Answer from the drawing. Dimensions are ordinates in mm from the lowest x, y and z of the part. A direction names the side the tool comes from. Coordinates: 2 decimals unless noted, no trailing zeros. Loops run counter-clockwise (first coordinate to the right, second up) from the corner with the lowest first, then second, coordinate; pieces in that order, holes last. Notation, with made-up numbers: M -0.5,4 L 9.5,4 A30 cw 9.5,34 Z; hole C -5,75.5 d8. An arc over 180 degrees is marked long. Put each result on its own line as item: value.
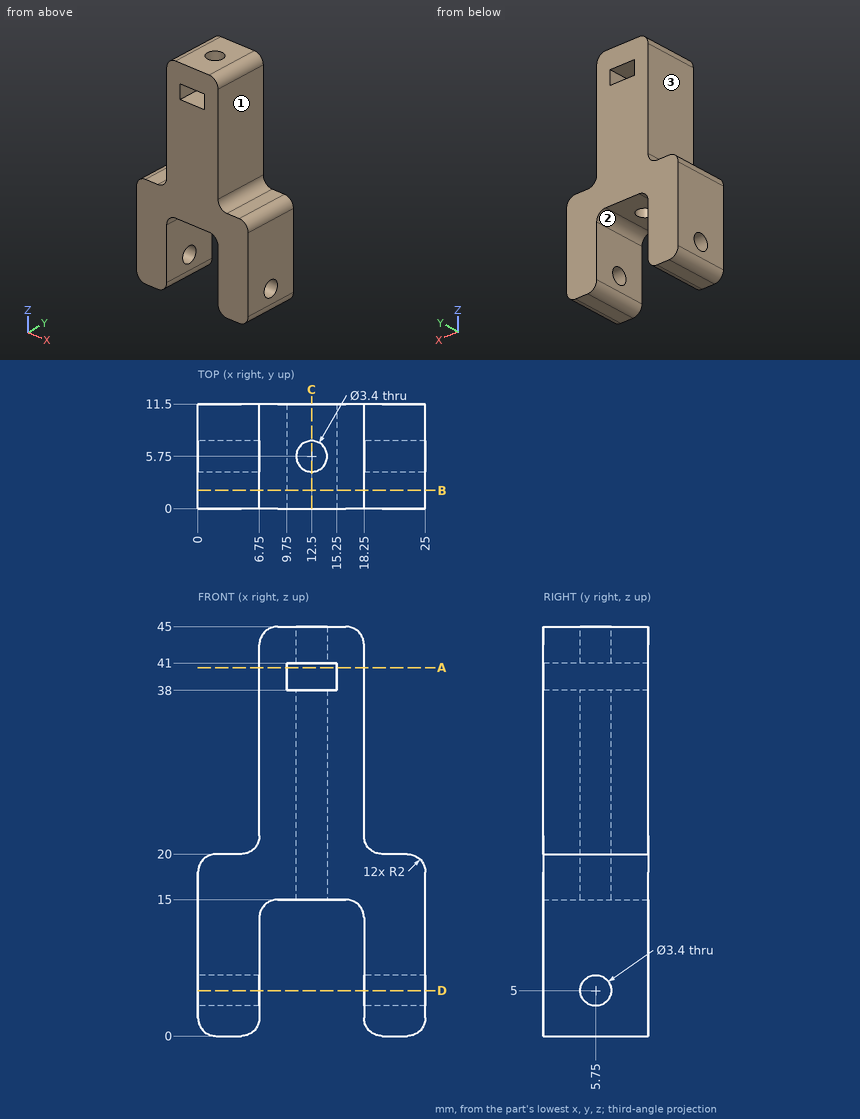
1) Find section B-B, the plane y = 2. Write down the section's boundary in (x, z).
Answer list:
outline: M 0,2 A2 ccw 2,0 L 4.75,0 A2 ccw 6.75,2 L 6.75,13 A2 cw 8.75,15 L 16.25,15 A2 cw 18.25,13 L 18.25,2 A2 ccw 20.25,0 L 23,0 A2 ccw 25,2 L 25,18 A2 ccw 23,20 L 20.25,20 A2 cw 18.25,22 L 18.25,43 A2 ccw 16.25,45 L 8.75,45 A2 ccw 6.75,43 L 6.75,22 A2 cw 4.75,20 L 2,20 A2 ccw 0,18 Z; hole M 9.75,38 L 15.25,38 L 15.25,41 L 9.75,41 Z
2) Given pin 1 Ø4.5 at (x, y) = (12.5, 5.75) entering from -Z; pin 2 Ø1.4 at (x, y) = (22, 3) entering from +Z; pin 3 Ø2.5 at (y, z) = (5, 40) entering from +X; pin 4 Ø3 at (y, z) = (5.75, 5) entering from -X, each flat-ended and moving along its own axis, determine where each tip first touches the part or whether it passes through.
Answer list:
pin 1: stops at z = 15
pin 2: stops at z = 20
pin 3: stops at x = 18.25
pin 4: passes through
3) Find section D-D, the plane z = 5. Write down the section's boundary in (x, y), plus the area to 3 significant figures.
Answer list:
outline: M 0,0 L 6.75,0 L 6.75,4.05 L 0,4.05 Z; M 0,7.45 L 6.75,7.45 L 6.75,11.5 L 0,11.5 Z; M 18.25,0 L 25,0 L 25,4.05 L 18.25,4.05 Z; M 18.25,7.45 L 25,7.45 L 25,11.5 L 18.25,11.5 Z
area: 109 mm^2
4) Find section C-C, the plane x = 12.5. Write down the section's boundary in (y, z), plus the area to 3 significant figures.
Answer list:
outline: M 0,15 L 4.05,15 L 4.05,38 L 0,38 Z; M 0,41 L 4.05,41 L 4.05,45 L 0,45 Z; M 7.45,15 L 11.5,15 L 11.5,38 L 7.45,38 Z; M 7.45,41 L 11.5,41 L 11.5,45 L 7.45,45 Z
area: 219 mm^2
5) Which of the six approach directions +Z, -Z, +X, -X, +Y, -Y give full straight-line access (tool end or side, diameter ignored) to the marked faces 1, 2 and 3?
Answer list:
face 1: +Z, +X, +Y, -Y
face 2: -Z, +Y, -Y
face 3: +Z, -X, +Y, -Y
6) Straight lines are drawn through the part: line 1 (X direction, y = 1, z = 3); line 2 (Y direction, x = 12.5, z = 43.4); line 3 (X direction, y = 6, z = 40). For each, find the intervals that lie inside material, in ascending order. Write a range as [from, to].
Answer list:
line 1: x = [0, 6.75], [18.25, 25]
line 2: y = [0, 4.05], [7.45, 11.5]
line 3: x = [6.75, 9.75], [15.25, 18.25]
7) Find section A-A, the plane z = 40.5. Write down the section's boundary in (x, y).
Answer list:
outline: M 6.75,0 L 9.75,0 L 9.75,11.5 L 6.75,11.5 Z; M 15.25,0 L 18.25,0 L 18.25,11.5 L 15.25,11.5 Z
